Source: CAD feature listing. Evaluate the final solid. Frame: model axes, mm. A direction names the side the tool comes from. Give positions to 0.01 mm unless a question says otherwise; leave off trailing zeros. Order: outer loops, then holes, each group sorted by start corner. A loop starts at its lowest first (then second) coordinate and runs counter-clockwise, first axis right, second up.
1) Draft query along X for faces 1 (the face through (0.28, 7.897, -5.07)), 2 (the face through (40, 22, -18)), 3 (the face through (1, 0, -5)). Return one class per face: released by +X, released by -X, zero draft, split by the parting line, or undercut.
2) Section D-D, the plane x = -32.5. Return loops of the section in (y, z).
3) Section B-B, the plane z = -18. Return loops of the section in (x, y), plus the area to 3 significant figures.
4) Material intervals for line 1 (Z direction, x = -28, y = 13); line 2 (X direction, y = 28.75, z = -26); line 3 (Y direction, x = 30, z = -12), sorted ascending.
5) Section A-A, the plane y = 16. Return loops of the section in (x, z).
6) First-contact query: P1, Ø6, axis at x = 8, y = 11.5, coming from the +Z side (3 decimals); P2, Ø7.5, axis at x = 28, z = -18.5, coming from the -Y side. Flat tips, straight axial feed; report the tip coordinate or a pass-through.
7) Access query for faces 4 (the face through (-40, 22, -18)), 5 (the face through (1, 10, -25)), 6 (the face through (0.3, 22.2, -30.1)). Directions: +Z, -Z, +X, -X, +Y, -Y. A direction counts if a zero-diameter tool reaches every point of the face in a straight line with its end or side. Return the directions, or none.
8) Section C-C, the plane x = 15. Return loops of the section in (y, z).
```python
from build123d import *

# Parameters (mm, degrees)
BOSS_EXTRUDE1_DEPTH = 40
CUT_EXTRUDE2_DEPTH  = 20


with BuildPart() as part:
    # Sketch1 → Boss-Extrude1 (new body, symmetric)
    with BuildSketch(Plane(origin=(0, 0, 0), x_dir=(0, 0, -1), z_dir=(1, 0, 0))):
        Polygon((0, 0), (0, 30), (35, 30), (35, 0), (25, 0), (25, 20), (10, 20), (10, 0), align=None)
    extrude(amount=BOSS_EXTRUDE1_DEPTH, both=True)

    # Sketch2 → Cut-Extrude2 (cut, symmetric)
    with BuildSketch(Plane(origin=(0, 0, 0), x_dir=(0, 0, -1), z_dir=(1, 0, 0))):
        Polygon((35, 25), (0, 5), (0, 30), (35, 30), align=None)
    extrude(amount=CUT_EXTRUDE2_DEPTH, both=True, mode=Mode.SUBTRACT)


solid = part.part
```
From the geometry:
1. face 1: undercut
1. face 2: released by +X
1. face 3: zero draft
2. outline: (0, -35) - (30, -35) - (30, 0) - (0, 0) - (0, -10) - (20, -10) - (20, -25) - (0, -25) - close
3. outline: (-40, 20) - (-20, 20) - (-20, 30) - (-40, 30) - close; (20, 20) - (40, 20) - (40, 30) - (20, 30) - close
3. area: 400 mm2
4. line 1: z = -35 to -25, -10 to 0
4. line 2: x = -40 to -20, 20 to 40
4. line 3: y = 20 to 30
5. outline: (-40, -35) - (40, -35) - (40, -25) - (-40, -25) - close; (-40, -10) - (-20, -10) - (-20, 0) - (-40, 0) - close; (20, -10) - (40, -10) - (40, 0) - (20, 0) - close
6. P1: stops at z = -6.125
6. P2: stops at y = 20
7. face 4: +Z, -Z, -X, +Y, -Y
7. face 5: +X, -X, -Y
7. face 6: +Z, +Y
8. outline: (0, -35) - (25, -35) - (19.29, -25) - (0, -25) - close; (0, -10) - (10.71, -10) - (5, 0) - (0, 0) - close
